For this review, use the dimensioned drawing (mm, ordinates from the lowest corner) and the shaded views. A direction names the side the tool comes from. Round coordinates to 2 decimals unless told otherwise and drop trailing zeros. Order: outer loops, then holes, each group sorted by start corner. A loop starts at its lowest first (then second) coordinate and runs counter-clockwise, first axis right, second up. Notation, with made-up numbers: M 52.5,89.5 L 92.5,89.5 A24 cw 92.5,111.5 Z; hole C 86.25,-6.75 d1. An arc over 180 degrees is marked long. Use a Markdown table: item, result. Add a question column.
1. For the marked faces 4 and 5, list the 3-axis set-ups (+Z, -Z, +X, -X, +Y, -Y) from which the entire face can be reached by the end or side of a thin tool; tool diameter is ignored.
2. Consider section A-A on y = 17. State the section outline as (x, z) points.
3. Consider section B-B on z = 16.5. State the section outline as (x, y) points.
4. To check wall thickness, follow probe 1 along Y at (x, z) = (13.5, 15.5); probe 2 along X at (y, z) = (23.5, 31); probe 3 along Y at (x, z) = (1, 16). State the ranges of each line that lie inside material, in increasing order.
5. The part is to be moulded in two halves that separate along Y. For the marked faces 1, 2 and 3, say which applies: +Y half, -Y half, draft (parallel to the pull), parting line (faces both ways), or undercut.
6. Consider section D-D on x = 8. State the section outline as (y, z) points, then the cut area to 3 significant figures.
7. Consider section C-C on x = 28. State the section outline as (y, z) points, then the cut area to 3 significant figures.
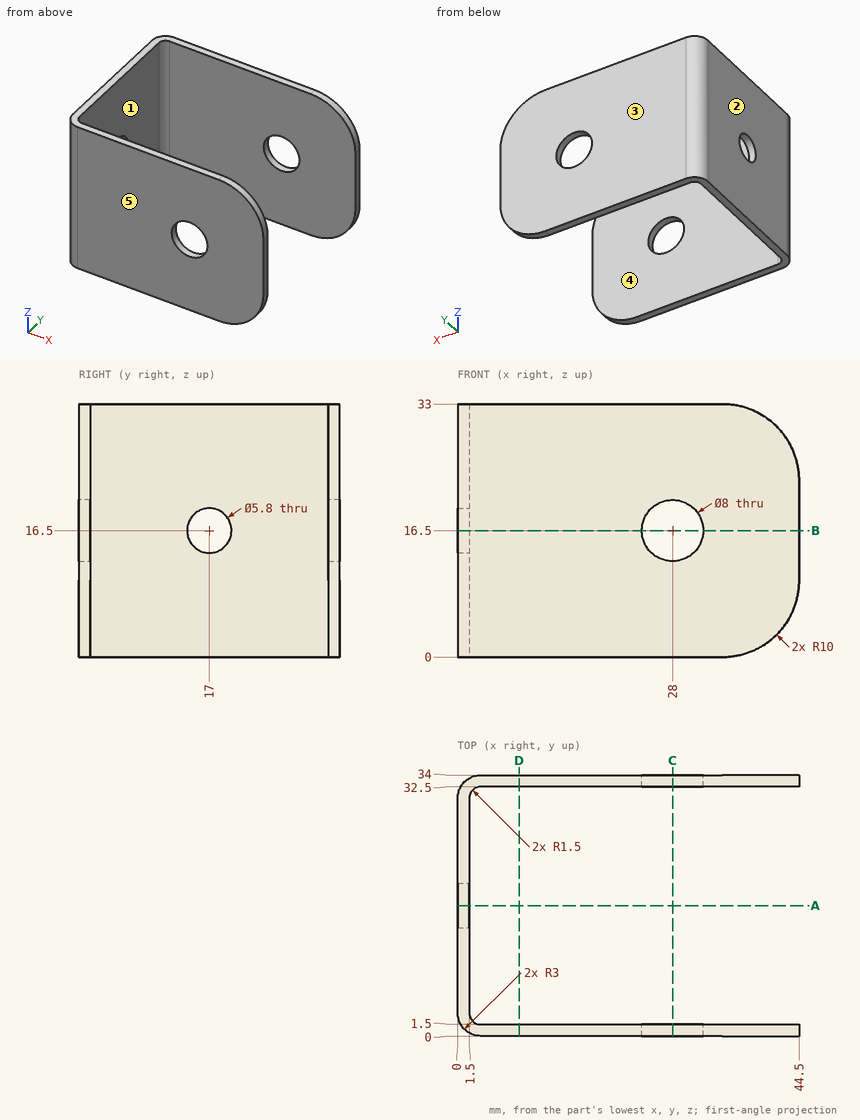
Answer block:
| question | item | result |
|---|---|---|
| 1 | face 4 | +Z, -Z, +X |
| 1 | face 5 | +Z, -Z, +X, -X, -Y |
| 2 | outline | M 0,0 L 1.5,0 L 1.5,13.6 L 0,13.6 Z; M 0,19.4 L 1.5,19.4 L 1.5,33 L 0,33 Z |
| 3 | outline | M 0,3 A3 ccw 3,0 L 24,0 L 24,1.5 L 3,1.5 A1.5 cw 1.5,3 L 1.5,14.1 L 0,14.1 Z; M 0,19.9 L 1.5,19.9 L 1.5,31 A1.5 cw 3,32.5 L 24,32.5 L 24,34 L 3,34 A3 ccw 0,31 Z; M 32,0 L 44.5,0 L 44.5,1.5 L 32,1.5 Z; M 32,32.5 L 44.5,32.5 L 44.5,34 L 32,34 Z |
| 4 | probe 1 | 0 to 1.5, 32.5 to 34 |
| 4 | probe 2 | 0 to 1.5 |
| 4 | probe 3 | 0.76 to 14.14, 19.86 to 33.24 |
| 5 | face 1 | undercut |
| 5 | face 2 | draft |
| 5 | face 3 | +Y half |
| 6 | outline | M 0,0 L 1.5,0 L 1.5,33 L 0,33 Z; M 32.5,0 L 34,0 L 34,33 L 32.5,33 Z |
| 6 | area | 99.0 mm^2 |
| 7 | outline | M 0,0 L 1.5,0 L 1.5,12.5 L 0,12.5 Z; M 0,20.5 L 1.5,20.5 L 1.5,33 L 0,33 Z; M 32.5,0 L 34,0 L 34,12.5 L 32.5,12.5 Z; M 32.5,20.5 L 34,20.5 L 34,33 L 32.5,33 Z |
| 7 | area | 75.0 mm^2 |
